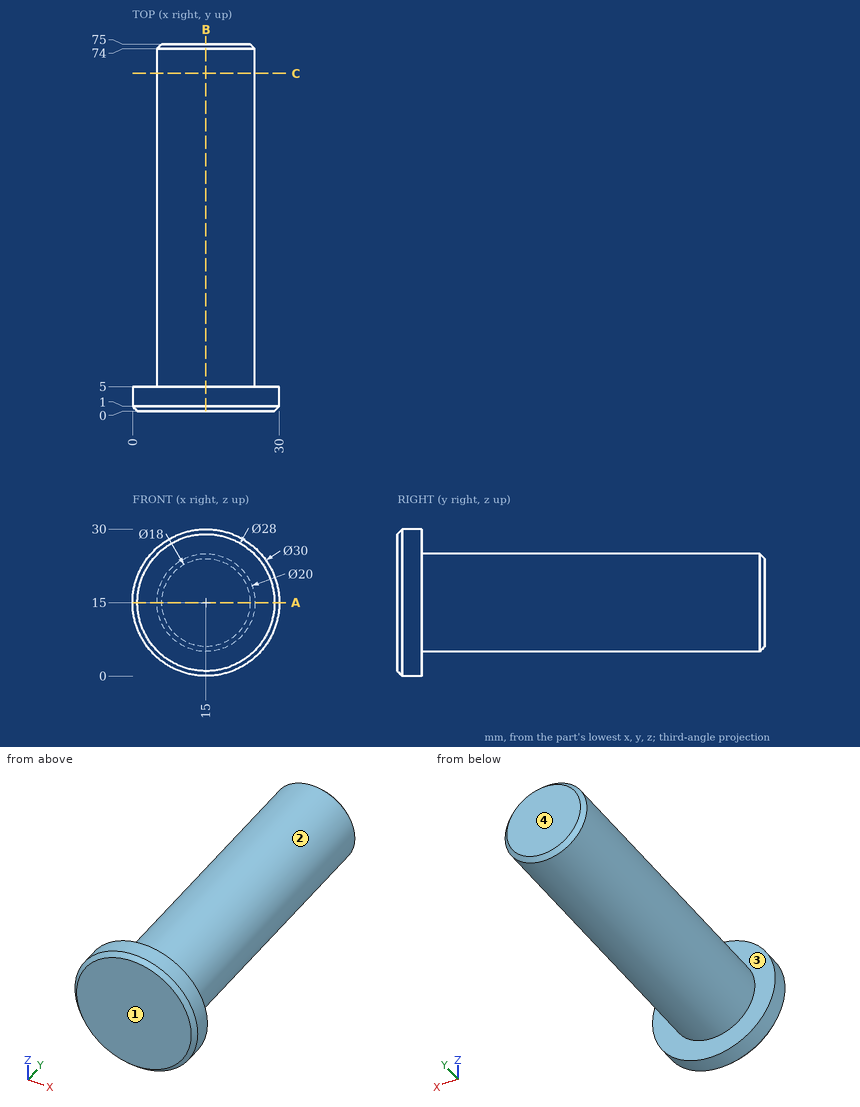
Geometry: see drawing. Coordinates: mm, zero at the bounding-box minimum. A direction names the side the tool comes from. Give positions to 0.01 mm unless a question says otherwise; leave off trailing zeros. Write each loop counter-clockwise with the first axis right and the second up, starting at its lowest first coordinate (ties: lowest second). Pieces come first, ordered by that corner, then holes. Notation, with made-up numbers: M 79.25,78.5 L 92.25,78.5 A17 ccw 92.25,99.5 Z; hole C 5,35 d1. An arc over 180 degrees is marked long. Return JSON: item names as keys, results as strings. Group by question number.
1) Cut plane A-A, the plane z = 15. Output: boundary loops of the cut face in (x, y), then the cut area to 3 significant figures.
2) Ray query, L1, parallel to Y at x = 10, z = 3; L2, parallel to Z at x = 18, y = 48.5; L3, parallel to Z at x = 22.5, y = 52. Return the intervals inside material, ascending.
3) Draft query along X for the marked faces 1 and 2. Return one class per face: released by +X, released by -X, zero draft, split by the parting line, or undercut.
4) First-contact query: pin 1 Ø10 at (y, z) = (39, 15) entering from -X; pin 2 Ø5 at (y, z) = (22, 6.5) entering from +X; pin 3 Ø12 at (x, y) = (6.5, 13.5) entering from +Z. Flat tips, straight axial feed; report the tip coordinate or a pass-through.
5) Cut plane B-B, the plane x = 15. Output: boundary loops of the cut face in (y, z), then the cut area to 3 significant figures.
6) Cut plane C-C, the plane y = 69. Output: boundary loops of the cut face in (x, z).
7) Set-up query: the marked faces 3 and 4. Return all of +Z, -Z, +X, -X, +Y, -Y with unobstructed straight access to the full face (end or side cutting, diameter ignored); none if empty.
Data:
{
 "1": {"outline": "M 0,1 L 1,0 L 29,0 L 30,1 L 30,5 L 25,5 L 25,74 L 24,75 L 6,75 L 5,74 L 5,5 L 0,5 Z", "area": "1,550 mm²"},
 "2": {"L1": "y = 0 to 5", "L2": "z = 5.46 to 24.54", "L3": "z = 8.39 to 21.61"},
 "3": {"face 1": "zero draft", "face 2": "split by the parting line"},
 "4": {"pin 1": "stops at x = 5", "pin 2": "stops at x = 23", "pin 3": "stops at z = 24.68"},
 "5": {"outline": "M 0,1 L 1,0 L 5,0 L 5,5 L 74,5 L 75,6 L 75,24 L 74,25 L 5,25 L 5,30 L 1,30 L 0,29 Z", "area": "1,550 mm²"},
 "6": {"outline": "C 15,15 d20"},
 "7": {"face 3": "+Y", "face 4": "+Z, -Z, +X, -X, +Y"}
}
